Source: three-view drawing plus pictorial views. Frame: mm from the lowest corner of the part. Coordinates: 2 decimals unless noted, no trailing zeros. Write each loop counter-clockwise with the first axis right and the second up, starting at its lowest first coordinate (ties: lowest second). Pieces come first, ordered by that corner, then holes. Notation, with made-up numbers: (40, 6) - (65, 6) arc R24 cw to (65, 45) - close; hole circle Ø3 at (9.25, 83.5). An arc over 180 degrees is marked (long way). Answer as a JSON object with one key per item and string values. Group by question number.
Item 1: Section C-C on x = 11.5. Return loops of the section in (y, z).
Item 2: First-contact query: pin 1 Ø4 at (x, y) = (10, 8) entering from -Z; pin 2 Ø3.5 at (y, z) = (9, 54.5) entering from +X; pin 3 Ø1.5 at (x, z) = (1.5, 97) entering from -Y; pin 4 Ø4 at (x, y) = (3, 3) entering from +Z. Flat tips, straight axial feed; report the tip coordinate or a pass-through.
Item 3: Section A-A on y = 3. Return loops of the section in (x, z).
Item 4: Line query: line 1 along Z through (x, y) = (0.75, 8.25); line 2 along Z through (x, y) = (1.5, 10.5); line 3 along X through (y, z) = (6.75, 55). Output: solid intervals per line, ascending. Write a range as from..to.
Item 5: Section B-B on z = 70.15. Return loops of the section in (x, y), and give its area (3 significant figures).
Item 6: Section D-D on z = 9.5. Return loops of the section in (x, y).
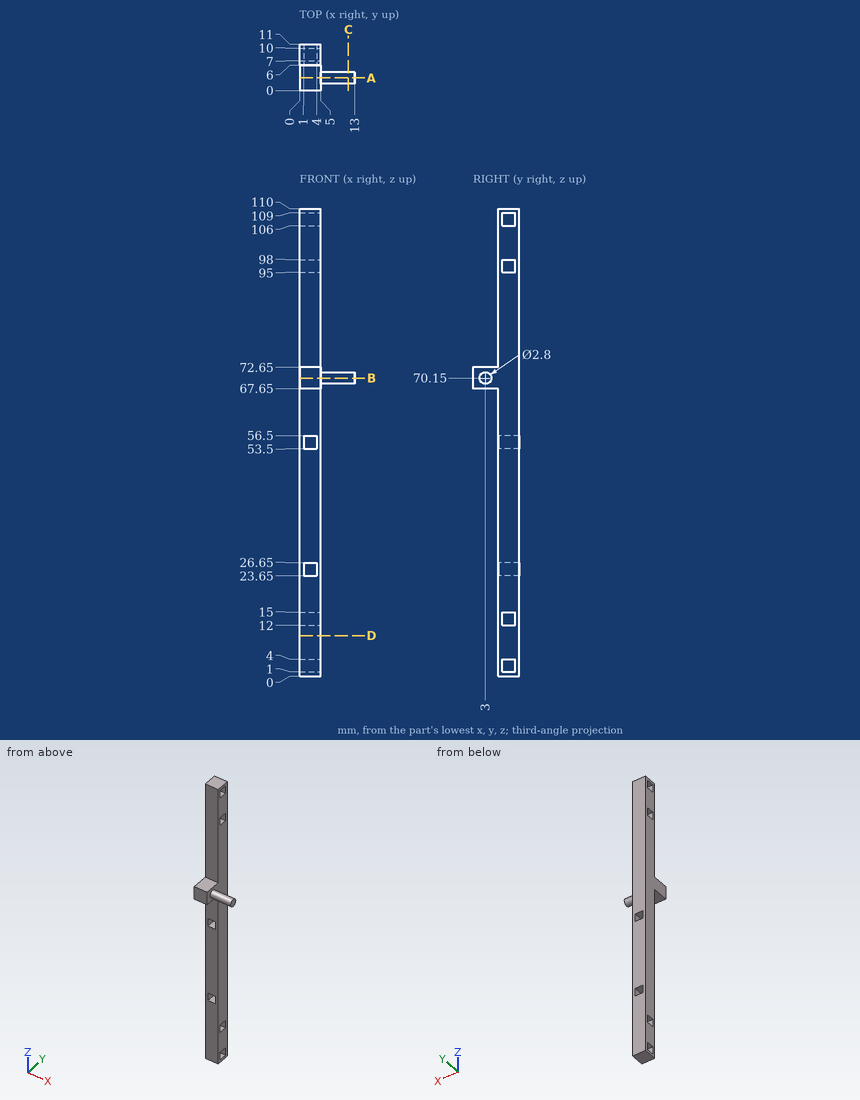
Checks:
{
 "1": {"outline": "circle Ø2.8 at (3, 70.15)"},
 "2": {"pin 1": "through", "pin 2": "x = 5", "pin 3": "y = 6", "pin 4": "z = 72.65"},
 "3": {"outline": "(0, 67.65) - (5, 67.65) - (5, 68.75) - (13, 68.75) - (13, 71.55) - (5, 71.55) - (5, 72.65) - (0, 72.65) - close"},
 "4": {"line 1": "0..1, 4..12, 15..95, 98..106, 109..110", "line 2": "0..23.65, 26.65..53.5, 56.5..110", "line 3": "0..1, 4..5"},
 "5": {"outline": "(0, 0) - (5, 0) - (5, 1.6) - (13, 1.6) - (13, 4.4) - (5, 4.4) - (5, 11) - (0, 11) - close", "area": "77.4 mm^2"},
 "6": {"outline": "(0, 6) - (5, 6) - (5, 11) - (0, 11) - close"}
}
